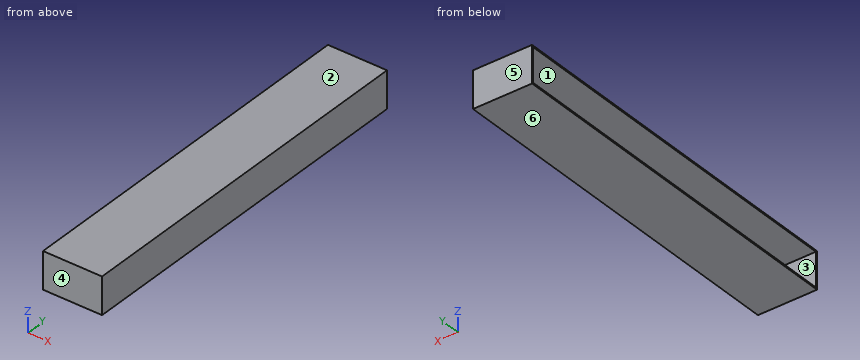
```python
from build123d import *

# Parameters (mm, degrees)
SKETCH_2_W        = 50
SKETCH_2_H        = 500
SKETCH_2_W_2      = 46
SKETCH_2_H_2      = 496
EXTRUDE_1_DEPTH   = 80
SKETCH_3_W        = 50
SKETCH_3_H        = 500
EXTRUDE_1_2_DEPTH = 2


with BuildPart() as part:
    # 草图2 → Extrude 1 (new body)
    with BuildSketch(Plane(origin=(-5, 0, 0), x_dir=(0, 0, -1), z_dir=(1, 0, 0))):
        with Locations((25, 225)):
            Rectangle(SKETCH_2_W, SKETCH_2_H)
        with Locations((25, 225)):
            Rectangle(SKETCH_2_W_2, SKETCH_2_H_2, mode=Mode.SUBTRACT)
    extrude(amount=EXTRUDE_1_DEPTH)

    # 草图3 → Extrude 1 2 (add)
    with BuildSketch(Plane(origin=(75, 0, 0), x_dir=(0, 0, -1), z_dir=(1, 0, 0))):
        with Locations((25, 225)):
            Rectangle(SKETCH_3_W, SKETCH_3_H)
    extrude(amount=-EXTRUDE_1_2_DEPTH)


solid = part.part
```
Source: CAD feature listing. Evaluate the final solid. Frame: model axes, mm. Face numbers are marked on the shaded views. A direction names the side the tool comes from. Coordinates: 2 decimals unless noted, no trailing zeros. Order: outer loops, then holes, each group sorted by start corner. A loop starts at its lowest first (then second) coordinate and runs counter-clockwise, first axis right, second up. Notation, with made-up numbers: M -31,-25.5 L -3,-25.5 A20 ccw -3,5.5 Z; hole C -38.5,87 d4. An arc over 180 degrees is marked long. Write each question's results on one line, items separated by ' | '. Start each with the question number.
1) Section query B-B (y = 309). Return the cut outline in (x, z).
2) Draft query along Y for the marked faces 3, 4, 5 and 6. Return one class per face: released by +Y, released by -Y, zero draft, split by the parting line, or undercut.
3) Section query A-A (x = 30.5). Return the cut outline in (y, z), plus the area to 3 significant figures.
4) Line query: line 1 (Z direction, x = 1.5, y = 225); line 2 (Y direction, x = 31.5, z = -11); line 3 (X direction, y = 202.5, z = -45.5). Output: solid intervals per line, ascending. Write a range as from..to.
5) Section query C-C (z = -17.5). Return the cut outline in (x, y).
6) Contact query for a flat-ended pin moving along its axis: pin 1 Ø6 at (y, z) = (101, -31) entering from -X. Output: stop coordinate, or through.
7) Access query for the marked faces 1 and 2. Directions: +Z, -Z, +X, -X, +Y, -Y. A direction counts if a zero-diameter tool reaches every point of the face in a straight line with its end or side. Return the directions, or none.
Answers:
1) outline: M -5,-50 L 75,-50 L 75,0 L -5,0 L -5,-2 L 73,-2 L 73,-48 L -5,-48 Z
2) face 3: undercut | face 4: released by -Y | face 5: released by +Y | face 6: zero draft
3) outline: M -25,-50 L 475,-50 L 475,0 L -25,0 Z; hole M -23,-48 L 473,-48 L 473,-2 L -23,-2 Z | area: 2,180 mm^2
4) line 1: z = -50..-48, -2..0 | line 2: y = -25..-23, 473..475 | line 3: x = 73..75
5) outline: M -5,-25 L 75,-25 L 75,475 L -5,475 L -5,473 L 73,473 L 73,-23 L -5,-23 Z
6) pin 1: stops at x = 73
7) face 1: -X | face 2: +Z, +X, -X, +Y, -Y
